```python
from build123d import *

# Parameters (mm, degrees)
F0_W     = 2
F0_H     = 12
F1_DEPTH = 45
F2_W     = 30
F2_H     = 20
F3_DEPTH = 14


with BuildPart() as f1:
    # F0 (on Right) → F1 (new body, symmetric)
    with BuildSketch(Plane.YZ):
        Polygon((48, 0), (0, 0), (0, -2), (50, -2), (50, 0), align=None)
        with Locations((49, 6)):
            Rectangle(F0_W, F0_H)
        Polygon((30, 12), (48, 12), (50, 12), (50, 14), (30, 14), align=None)
    extrude(amount=F1_DEPTH, both=True)

    # F2 (on face) → F3 (cut)
    with BuildSketch(Plane.XY.offset(14)):
        with Locations((0, 40)):
            Rectangle(F2_W, F2_H)
    extrude(amount=-F3_DEPTH, mode=Mode.SUBTRACT)


solid = f1.part
```
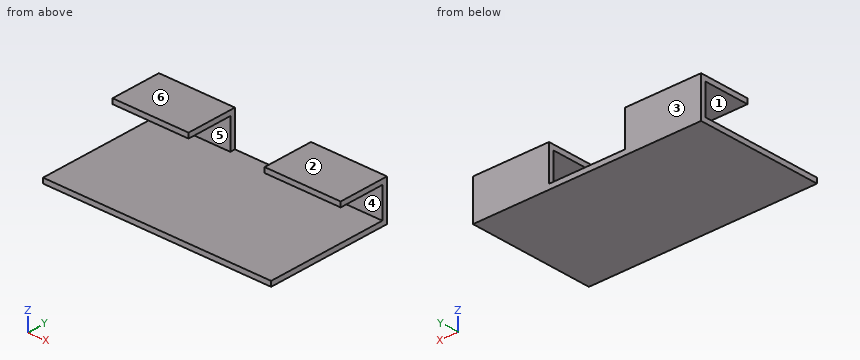
Geometry: final body of the model. Coordinates: model frame, mm. Face numbers are marked on the shaded views. A direction names the side the tool comes from. Give positions to 0.01 mm unless a question says otherwise; leave off trailing zeros. Loops run counter-clockwise (first coordinate to the right, second up) from the corner with the lowest first, then second, coordinate; pieces in that order, holes last. Notation, with made-up numbers: (43.5, 82) - (82.5, 82) arc R23 cw to (82.5, 110) - close; hole circle Ø5 at (-31, 40). An arc over 180 degrees is marked (long way). Answer as CSV lines item,"result". Start each with the question number.
(1) Reachability of the marked faces 5 and 6 from +Z, -Z, +X, -X, +Y, -Y: full face, straight path, thin tool, end or side. Return the list, or none.
(2) Section query B-B (y = 36.5). Output: boundary loops of the cut face in (x, z), and give its area (3 significant figures).
(3) Section query D-D (y = 27). Output: boundary loops of the cut face in (x, z).
(4) Pin query (flat end, axial travel): P1, Ø1, axis at x = 29, z = 10, coming from the -Y side; P2, Ø1.6, axis at x = 32.5, z = 12.5, coming from the -Y side; P3, Ø25, axis at x = 0, y = 13, coming from the +Z side. Return the tip coordinate at first contact, or that it passes through.
(5) Mould query, pull axis Z, two halves, no side actions, for the marked faces 1, 2, 3 and 4. Classes: +Z half, -Z half, draft (parallel to the pull), parting line (faces both ways), or undercut.
(6) Section query A-A (z = 7). Output: boundary loops of the cut face in (x, y).
(7) Section query C-C (x = 29.5). Output: boundary loops of the cut face in (y, z).
(8) Ray query, line 1 along Z through (x, y) = (29, 33); line 2 along Y through (x, z) = (29.5, 11.5); line 3 along Z through (x, y) = (-36.5, 9). Return the intervals inside material, ascending. Write a range as [from, to].
Worked answers:
1,face 5,"+X, -X, -Y"
1,face 6,"+Z, +X, -X, +Y, -Y"
2,outline,"(-45, -2) - (45, -2) - (45, 0) - (-45, 0) - close; (-45, 12) - (-15, 12) - (-15, 14) - (-45, 14) - close; (15, 12) - (45, 12) - (45, 14) - (15, 14) - close"
2,area,"300 mm^2"
3,outline,"(-45, -2) - (45, -2) - (45, 0) - (-45, 0) - close"
4,P1,"stops at y = 48"
4,P2,"stops at y = 30"
4,P3,"stops at z = 0"
5,face 1,"undercut"
5,face 2,"+Z half"
5,face 3,"draft"
5,face 4,"undercut"
6,outline,"(-45, 48) - (-15, 48) - (-15, 50) - (-45, 50) - close; (15, 48) - (45, 48) - (45, 50) - (15, 50) - close"
7,outline,"(0, -2) - (50, -2) - (50, 14) - (30, 14) - (30, 12) - (48, 12) - (48, 0) - (0, 0) - close"
8,line 1,"z = [-2, 0], [12, 14]"
8,line 2,"y = [48, 50]"
8,line 3,"z = [-2, 0]"
